Job drawing, mm, ordinate dimensions from the low corner. One solid piece. Round coordinates to 2 decimals unless told otherwise and drop trailing zeros. Write each loop counter-clockwise with the first axis right and the second up, starting at its lowest first coordinate (ties: lowest second). Pieces come first, ordered by that corner, then holes. Notation, with made-up numbers: M -35.5,69 L 9.5,69 A11 ccw 9.5,88 Z; hole C -18.75,76 d9. An arc over 180 degrees is marked long. Write each question's results on one line, items separated by ' | '. Start each with the question number.
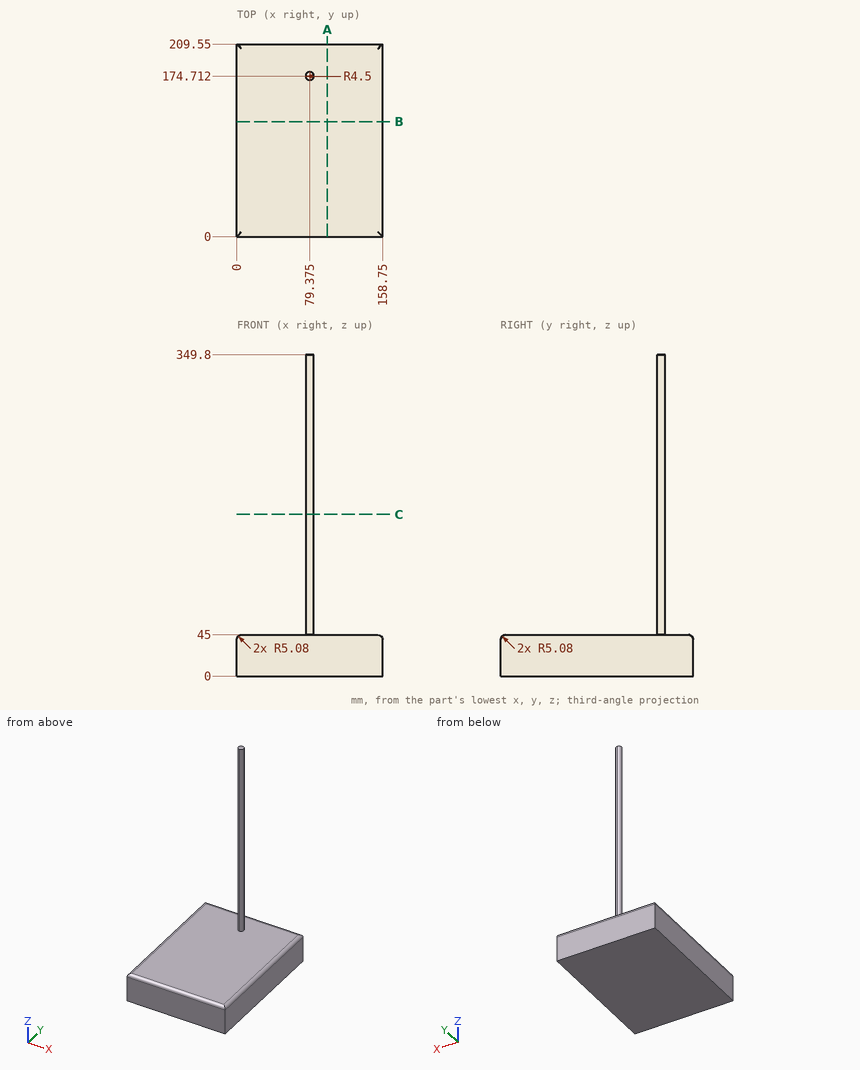
1) Drop flat-ended pins along their axis: pin 1 Ø8 at (x, y) = (34, 35.5) entering from +Z; pin 2 Ø2 at (y, z) = (168.5, 303.5) entering from +X; pin 3 Ø6 at (x, y) = (109.5, 112.5) entering from -Z. Give the stop position or say it passes through.
2) Saw through at C-C, the plane z = 176. Write the cut outline in (x, y) (1 decimal).
3) Saw through at A-A, the plane x = 98.5. Write the cut outline in (y, z), plus the area to 3 significant figures.
4) Saw through at B-B, the plane y = 125. Write the cut outline in (x, z), plus the area to 3 significant figures.
5) Wall check: line 1 along Z through (x, y) = (97, 144.5); line 2 along Y through (x, z) = (78, 73.5). Give the ranges that are in metal, low to high. Write a range as from..to.
Filled sheet:
1) pin 1: stops at z = 45 | pin 2: passes through | pin 3: stops at z = 0
2) outline: C 79.4,174.7 d9
3) outline: M 0,0 L 209.55,0 L 209.55,39.92 A5.08 ccw 204.47,45 L 5.08,45 A5.08 ccw 0,39.92 Z | area: 9,420 mm^2
4) outline: M 0,0 L 158.75,0 L 158.75,39.92 A5.08 ccw 153.67,45 L 5.08,45 A5.08 ccw 0,39.92 Z | area: 7,130 mm^2
5) line 1: z = 0..45 | line 2: y = 170.43..179
